Verification items for the finished model (mm, model axes). A direction names the side the tool comes from. Give positions to 0.01 mm unless a question says otherwise; leave off trailing zeros. Write each loop counter-clockwise with the first axis right and the second up, starting at its lowest first coordinate (ties: lowest second). Pieces come first, ordered by that corner, then holes. Notation, with made-up numbers: (-17.75, 47.5) -> (32.25, 47.5) arc R17 cw to (32.25, 68.5) -> close; hole circle Ø8 at (-29.75, -4.5). An arc over 180 degrees is marked (long way). Answer as CSV lines item,"result". Start each with the question number.
1) Gauge pin test, flat end, axial feed: pin 1 Ø9 at (x, y) = (0, -4) entering from +Z. Record the tip position at first contact, or that the pin passes through.
2) Sectioned sample at B-B on z = 12. Record the cut outline in (x, y).
3) Mould release check, pull along Y, two halves, no side actions. Record for faces 4 (the cylindrical face through (24.51, 0.42, -0.35)), 5 (the flat face through (-1, 4, -25)), 6 (the conical face through (-19.7, 2.7, -3.9)): released by +Y, released by -Y, zero draft, split by the parting line, or undercut.
4) Material ranges on L1, parallel to Y at x = 0, z = 21; L2, parallel to Z at x = 20, y = 6.5; L3, parallel to X at y = -1.25, z = 13.5, recorded low to high.
5) Sectioned sample at C-C on z = -15. Record the cut outline in (x, y), and give its area (3 significant figures).
6) Tool access check on faces 1 (the cylindrical face through (-18.69, 9.17, -3)), 2 (the cylindrical face through (-6.55, -3.94, 17.23)), 3 (the flat face through (52.5, 0, 0)). Record the directions out of +Z, -Z, +X, -X, +Y, -Y that give a thin tool (end or side, any length) a straight path to the whole face; none if there is none.
7) Sectioned sample at D-D on z = 20. Record the cut outline in (x, y).
8) Sectioned sample at A-A on x = -34. Record the cut outline in (y, z).
```python
from build123d import *

# Parameters (mm, degrees)
ESBO_O1_W                             = 105
ESBO_O1_H                             = 30
ESBO_O1_R                             = 9.5
ESBO_O1_R_2                           = 4.25
RESSALTO_EXTRUS_O1_DEPTH              = 25
M4X0_7_TAPPED_HOLE1_D                 = 3.3
M4X0_7_TAPPED_HOLE1_DEPTH             = 11.5
M4X0_7_TAPPED_HOLE1_TIP               = 0.991420021
ESBO_O4_R                             = 5.1
CORTE_EXTRUS_O1_DEPTH                 = 11
FURO_ROSCADO_DE_M3_5X0_62_D           = 2.9
FURO_ROSCADO_DE_M3_5X0_62_DEPTH       = 15
FURO_ROSCADO_DE_M3_5X0_62_CSINK_D     = 3.55
FURO_ROSCADO_DE_M3_5X0_62_CSINK_ANGLE = 90
FURO_ROSCADO_DE_M3_5X0_62_TIP         = 0.871247898


with BuildPart() as part:
    # Esboço1 → Ressalto-extrusão1 (new, symmetric)
    with BuildSketch(Plane.XY):
        Rectangle(ESBO_O1_W, ESBO_O1_H)
        with Locations((-34, 0)):
            Circle(ESBO_O1_R, mode=Mode.SUBTRACT)
        with Locations((34, 0)):
            Circle(ESBO_O1_R, mode=Mode.SUBTRACT)
        with Locations((0, -4)):
            Circle(ESBO_O1_R_2, mode=Mode.SUBTRACT)
    extrude(amount=RESSALTO_EXTRUS_O1_DEPTH, both=True)

    # M4x0.7 Tapped Hole1
    with Locations(Plane(origin=(0, 15, 0), x_dir=(1, 0, 0), z_dir=(0, 1, 0))):
        with Locations((20, 19), (20, 4), (-20, 4), (-20, 19)):
            Hole(M4X0_7_TAPPED_HOLE1_D / 2, depth=M4X0_7_TAPPED_HOLE1_DEPTH)
            with Locations((0, 0, -(M4X0_7_TAPPED_HOLE1_DEPTH + M4X0_7_TAPPED_HOLE1_TIP / 2))):  # 118° drill point
                Cone(0, M4X0_7_TAPPED_HOLE1_D / 2, M4X0_7_TAPPED_HOLE1_TIP, mode=Mode.SUBTRACT)

    # Esboço4 → Corte-extrusão1 (cut)
    with BuildSketch(Plane.XY.offset(25)):
        with Locations((0, -4)):
            Circle(ESBO_O4_R)
    extrude(amount=-CORTE_EXTRUS_O1_DEPTH, mode=Mode.SUBTRACT)

    # Furo roscado de M3.5x0.62
    with Locations(Plane.XY.offset(25)):
        with Locations((-8, -4), (0, 4), (8, -4), (0, -12)):
            CounterSinkHole(FURO_ROSCADO_DE_M3_5X0_62_D / 2, FURO_ROSCADO_DE_M3_5X0_62_CSINK_D / 2, depth=FURO_ROSCADO_DE_M3_5X0_62_DEPTH, counter_sink_angle=FURO_ROSCADO_DE_M3_5X0_62_CSINK_ANGLE)
            with Locations((0, 0, -(FURO_ROSCADO_DE_M3_5X0_62_DEPTH + FURO_ROSCADO_DE_M3_5X0_62_TIP / 2))):  # 118° drill point
                Cone(0, FURO_ROSCADO_DE_M3_5X0_62_D / 2, FURO_ROSCADO_DE_M3_5X0_62_TIP, mode=Mode.SUBTRACT)


solid = part.part
```
Ans:
1,pin 1,"stops at z = 14"
2,outline,"(-52.5, -15) -> (52.5, -15) -> (52.5, 15) -> (-52.5, 15) -> close; hole circle Ø19 at (-34, 0); hole circle Ø2.9 at (-8, -4); hole circle Ø8.5 at (0, -4); hole circle Ø2.9 at (0, -12); hole circle Ø2.9 at (0, 4); hole circle Ø2.9 at (8, -4); hole circle Ø19 at (34, 0)"
3,face 4,"undercut"
3,face 5,"zero draft"
3,face 6,"released by +Y"
4,L1,"y = -15 to -13.45, -10.55 to -9.1, 1.1 to 2.55, 5.45 to 15"
4,L2,"z = -25 to -20.65, -17.35 to -5.65, -2.35 to 25"
4,L3,"x = -52.5 to -43.42, -24.58 to -3.24, 3.24 to 24.58, 43.42 to 52.5"
5,outline,"(-52.5, -15) -> (52.5, -15) -> (52.5, 15) -> (-52.5, 15) -> close; hole circle Ø19 at (-34, 0); hole circle Ø8.5 at (0, -4); hole circle Ø19 at (34, 0)"
5,area,"2,530 mm²"
6,face 1,"+Y"
6,face 2,"+Z"
6,face 3,"+Z, -Z, +X, +Y, -Y"
7,outline,"(-52.5, -15) -> (52.5, -15) -> (52.5, 15) -> (-52.5, 15) -> close; hole circle Ø19 at (-34, 0); hole circle Ø2.9 at (-8, -4); hole circle Ø10.2 at (0, -4); hole circle Ø2.9 at (0, -12); hole circle Ø2.9 at (0, 4); hole circle Ø2.9 at (8, -4); hole circle Ø19 at (34, 0)"
8,outline,"(-15, -25) -> (-9.5, -25) -> (-9.5, 25) -> (-15, 25) -> close; (9.5, -25) -> (15, -25) -> (15, 25) -> (9.5, 25) -> close"
